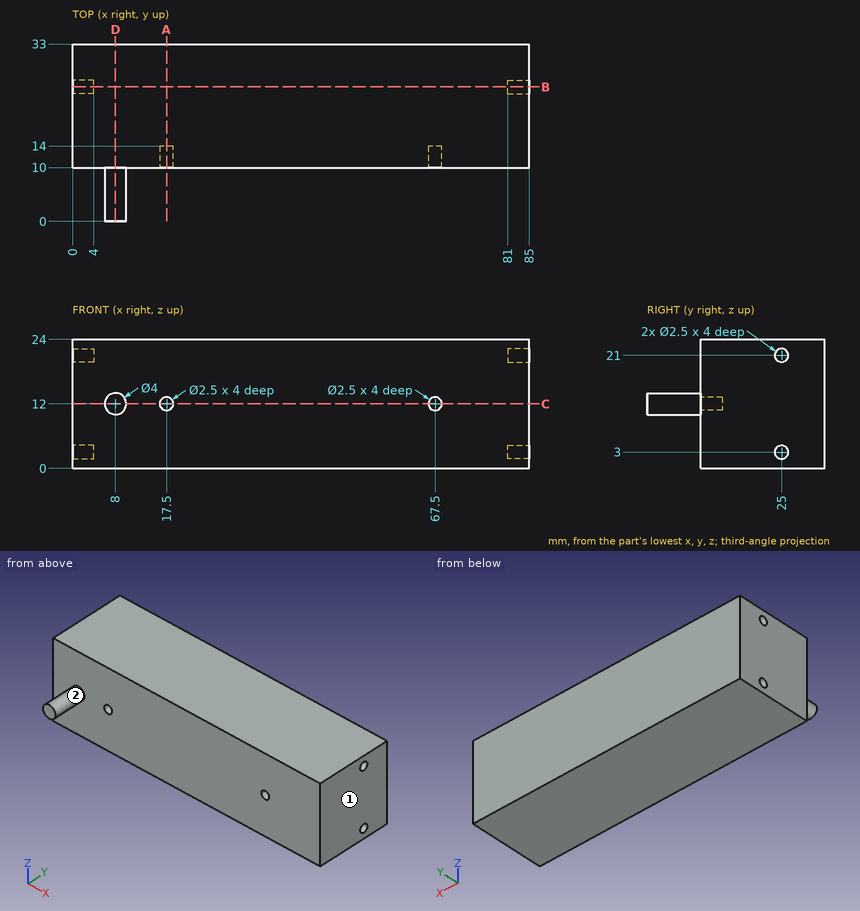
The figure shows three views and two pictorial views of one solid part (mm, origin at its lowest corner). Answer the questions. A direction names the side the tool comes from. Coordinates: 2 decimals unless noted, no trailing zeros. Order: outer loops, then holes, each group sorted by start corner. A loop starts at its lowest first (then second) coordinate and runs counter-clockwise, first axis right, second up. Notation, with made-up numbers: (9, -15.5) - (32, -15.5) arc R37 cw to (32, 22.5) - close; hole circle Ø7 at (-12, -1.5). An arc over 180 degrees is marked (long way). Answer as a JSON object with one key per item and string values.
1. Find section B-B on y = 25. Determine the outline of the cut face in (x, z).
Output values:
{"outline": "(0, 0) - (85, 0) - (85, 1.75) - (81, 1.75) - (81, 4.25) - (85, 4.25) - (85, 19.75) - (81, 19.75) - (81, 22.25) - (85, 22.25) - (85, 24) - (0, 24) - (0, 22.25) - (4, 22.25) - (4, 19.75) - (0, 19.75) - (0, 4.25) - (4, 4.25) - (4, 1.75) - (0, 1.75) - close"}
2. Each of these flat-tipped pins is pushed along its axis until it touches: P1, Ø5, axis at x = 17.5, z = 4, coming from the -Y side; P2, Ø1.5, axis at y = 25, z = 3, coming from the +X side; P3, Ø2, axis at y = 25, z = 21, coming from the -X side. Where does it stop, or does it pass through?
Output values:
{"P1": "stops at y = 10", "P2": "stops at x = 81", "P3": "stops at x = 4"}
3. Consider line 1 (Y direction, x = 83.6, z = 21); line 2 (Z direction, x = 17.5, y = 11.2); line 3 (X direction, y = 25.5, z = 21.75). Determine where each line is inside the solid, lowest interval first.
Output values:
{"line 1": "y = 10 to 23.75, 26.25 to 33", "line 2": "z = 0 to 10.75, 13.25 to 24", "line 3": "x = 4 to 81"}
4. Find section A-A on x = 17.5. Determine the outline of the cut face in (y, z), plus the area to 3 significant figures.
Output values:
{"outline": "(10, 0) - (33, 0) - (33, 24) - (10, 24) - (10, 13.25) - (14, 13.25) - (14, 10.75) - (10, 10.75) - close", "area": "542 mm²"}
5. Find section D-D on x = 8. Determine the outline of the cut face in (y, z).
Output values:
{"outline": "(0, 10) - (10, 10) - (10, 0) - (33, 0) - (33, 24) - (10, 24) - (10, 14) - (0, 14) - close"}
6. A tool of negligible diameter and unlimited length cuts with its end or side. For the marked faces 1 and 2, from which of +Z, -Z, +X, -X, +Y, -Y can it reach the whole face along a straight path? Write none if from no direction.
Output values:
{"face 1": "+Z, -Z, +X, +Y, -Y", "face 2": "-Y"}
7. Find section C-C on z = 12. Determine the outline of the cut face in (x, y).
Output values:
{"outline": "(0, 10) - (6, 10) - (6, 0) - (10, 0) - (10, 10) - (16.25, 10) - (16.25, 14) - (18.75, 14) - (18.75, 10) - (66.25, 10) - (66.25, 14) - (68.75, 14) - (68.75, 10) - (85, 10) - (85, 33) - (0, 33) - close"}
